Can you work these out from the model? Positions are in its coordinate system, mm. A direction names the side the tool comes from. Coordinates: 2 decimals unless noted, no trailing zeros. Loops run counter-clockwise (first coordinate to the right, second up) from the corner with the lowest first, then second, coordinate; pieces in that order, holes last.
```python
from build123d import *

# Parameters (mm, degrees)
F0_R     = 4
F1_DEPTH = 64
F2_DEPTH = 64
F3_W     = 0.5
F3_H     = 62
F4_DEPTH = 25


with BuildPart() as f1:
    # F0 (on Top) → F1 (new body)
    with BuildSketch(Plane.XY):
        with BuildLine():
            ThreePointArc((0, -6), (4.242641, -4.242641), (6, 0))
            ThreePointArc((6, 0), (-4.242641, 4.242641), (0, -6))
        make_face()
        Circle(F0_R, mode=Mode.SUBTRACT)
    extrude(amount=F1_DEPTH)

    # F0 (on Top) → F2 (join)
    with BuildSketch(Plane.XY):
        with BuildLine():
            Line((8, 0), (6, 0))
            ThreePointArc((6, 0), (4.242641, -4.242641), (0, -6))
            ThreePointArc((0, -6), (4.274303, -5.189002), (7.626499, -2.415889))
            ThreePointArc((7.626499, -2.415889), (7.906073, -1.222295), (8, 0))
        make_face()
    extrude(amount=F2_DEPTH)

    # F3 (on face) → F4 (cut)
    with BuildSketch(Plane(origin=(0, 0, 0), x_dir=(-1, 0, 0), z_dir=(0, 1, 0))):
        with Locations((-7.25, 32.5)):
            Rectangle(F3_W, F3_H)
    extrude(amount=-F4_DEPTH, mode=Mode.SUBTRACT)


solid = f1.part
```
(1) I'm going to push flat-ended pins straight in: pin 1 (0.8 mm diameter, centred on y = -1.5, z = 32, fed in from -X); pin 2 (1.6 mm diameter, centred on y = -1, z = 35, fed in from +X); pin 3 (1 mm diameter, centred on x = 6, y = 4.5, fed in from +Z); pin 4 (3 mm diameter, centred on y = -3.5, z = 11.5, fed in from +X). Where does each tip first touch, or does it pass through?
Check values:
pin 1: stops at x = -5.9
pin 2: stops at x = 8
pin 3: passes through
pin 4: stops at x = 7.75
(2) If we mould it in two halves opening along Z, with no side actions, what happens to faces 1 (the flat face through (4, -1.3, 0)), 2 (the cylindrical face through (-4.1, 4.38, 31.55)), 3 (the flat face through (7.5, -1, 32))? For each: released by +Z, released by -Z, zero draft, split by the parting line, or undercut.
Check values:
face 1: released by -Z
face 2: zero draft
face 3: undercut
(3) I want a section at D-D on x = 3. Write out the boundary of the cut face in (y, z).
Check values:
outline: (-5.67, 0) - (-2.65, 0) - (-2.65, 64) - (-5.67, 64) - close; (2.65, 0) - (5.2, 0) - (5.2, 64) - (2.65, 64) - close
(4) I want a section at B-B on y = -1.5. Write out the boundary of the cut face in (x, z).
Check values:
outline: (-5.81, 0) - (-3.71, 0) - (-3.71, 64) - (-5.81, 64) - close; (3.71, 0) - (7.86, 0) - (7.86, 64) - (3.71, 64) - close; hole (7, 1.5) - (7.5, 1.5) - (7.5, 63.5) - (7, 63.5) - close
(5) If I drill on probe 1 along Y at (x, z) = (0, 38.5); probe 2 along X at (y, z) = (-1.5, 9); probe 3 along X at (y, z) = (3.25, 50), over which ranges is the centre line in solid material (lowest first)?
Check values:
probe 1: y = -6 to -4, 4 to 6
probe 2: x = -5.81 to -3.71, 3.71 to 7, 7.5 to 7.86
probe 3: x = -5.04 to -2.33, 2.33 to 5.04
(6) Which directions (+Z, -Z, +X, -X, +Y, -Y) give clear straight access to the entire face, cutting with the end or side of a thin tool? Please do faces 4 (the cylindrical face through (3.31, -5.574, 31.552)), 5 (the flat face through (6.8, 0, 31.6)), 6 (the flat face through (7, -2, 32)).
Check values:
face 4: +Z, -Z, -Y
face 5: +Z, -Z, +X, +Y
face 6: +Y, -Y
(7) I want a section at A-A on z = 51. Write out the boundary of the cut face in (x, y), then the cut area to 3 significant figures.
Check values:
outline: (0, -6) arc R8.73 ccw to (7, -3.18) - (7, 0) - (6, 0) arc R6 ccw (long way) to start; (7.5, -2.59) arc R8.73 ccw to (7.63, -2.42) arc R8 ccw to (8, 0) - (7.5, 0) - close; hole circle Ø8 at (0, 0)
area: 72.0 mm2
(8) I want a section at C-C on x = -3. Write out the boundary of the cut face in (y, z), then the cut area to 3 significant figures.
Check values:
outline: (-5.2, 0) - (-2.65, 0) - (-2.65, 64) - (-5.2, 64) - close; (2.65, 0) - (5.2, 0) - (5.2, 64) - (2.65, 64) - close
area: 326 mm2
